Design review of the part built by this model. Coordinates are the model's own, in mm. Face numbers are marked on the shaded views. A direction names the side the tool comes from. Give positions to 0.01 mm unless a question says otherwise; leave off trailing zeros. Write each loop counter-clockwise with the first axis right and the second up, starting at its lowest first coordinate (ties: lowest second). Pieces come first, ordered by that corner, then holes. Notation, with made-up numbers: M 23,-9 L 45,-9 A31 cw 45,30 Z; hole C 83,-25 d6. An arc over 180 degrees is marked long. Use a Markdown table: item, result. Add a question column.
Autodesk Inventor part; units mm, degrees
ref_plane "YZ Plane" through (0, 0, 0) normal (1, 0, 0) x (0, 1, 0)
ref_plane "XZ Plane" through (0, 0, 0) normal (0, 1, 0) x (-1, 0, 0)
ref_plane "XY Plane" through (0, 0, 0) normal (0, 0, 1) x (1, 0, 0)
sketch "Sketch1" plane through (0, 0, 0) normal (0, 1, 0) x (-1, 0, 0)
  line L0 (0, 0) -> (19.1, 0)
  line L1 (19.1, 0) -> (19.1, -10)
  line L2 (19.1, -10) -> (0, -10)
  line L3 (0, -10) -> (0, 0)
  line L4 (12.55, -10) -> (6.55, -10)
  line L5 (6.55, -10) -> (6.55, -6)
  line L6 (6.55, -6) -> (12.55, -6)
  line L7 (12.55, -6) -> (12.55, -10)
  line L8 (0, 0) -> (-6, 0)
  line L9 (-6, 0) -> (-6, -17)
  line L10 (-6, -17) -> (0, -17)
  line L11 (0, -17) -> (0, 0)
  line L12 (19.1, 0) -> (25.1, 0)
  line L13 (25.1, 0) -> (25.1, -17)
  line L14 (25.1, -17) -> (19.1, -17)
  line L15 (19.1, -17) -> (19.1, 0)
  point P0 (9.55, -6)
  point P1 (9.55, 0)
  point P2 (6.55, -10)
  point P3 (0, -10)
  dimension "d0" = 6
  dimension "d1" = 19.1
  dimension "d2" = 4
  dimension "d3" = 10
  dimension "d6" = 6
  dimension "d7" = 6
  dimension "d8" = 17
  dimension "d20" = 7
extrude "Extrusion1" add sketch "Sketch1" along normal blind 10 contours L0 L1 L2 L7 L6 L5 L3 | L3 L11 L10 L9 L8 | L12 L13 L14 L15 L1
sketch "Sketch2" plane through (0, 0, 0) normal (0, -1, 0) x (1, 0, 0)
  line L0 (-25.1, 0) -> (6, 0)
  line L1 (-25.1, -17) -> (-25.1, 0)
  line L2 (-19.1, -17) -> (-25.1, -17)
  line L3 (-19.1, -10) -> (-19.1, -17)
  line L4 (-12.55, -10) -> (-19.1, -10)
  line L5 (-12.55, -6) -> (-12.55, -10)
  line L6 (-6.55, -6) -> (-12.55, -6)
  line L7 (-6.55, -10) -> (-6.55, -6)
  line L8 (0, -10) -> (-6.55, -10)
  line L9 (0, -17) -> (0, -10)
  line L10 (6, -17) -> (0, -17)
  line L11 (6, 0) -> (6, -17)
  line L12 (6, -17) -> (16, -17)
  line L13 (16, -17) -> (16, 10)
  line L14 (16, 10) -> (-35.1, 10)
  line L15 (-35.1, 10) -> (-35.1, -17)
  line L16 (-35.1, -17) -> (-25.1, -17)
  point P0 (0, 0)
  dimension "d9" = 10
  dimension "d10" = 10
  dimension "d11" = 10
extrude "Extrusion2" add sketch "Sketch2" against normal blind 2 contours L1 L16 L15 L14 L13 L12 L11 L0
chamfer "Chamfer1" distance 2 angle 45 7 edges at (-19.1, 10, -13.5) (-15.825, 10, -10) (-9.55, 10, -6) (-6.55, 10, -8) (0, 10, -13.5) (-3.275, 10, -10) (-12.55, 10, -8)
chamfer "Chamfer2" distance 2 angle 45 3 edges at (6, 10, -8.5) (-9.55, 10, 0) (-25.1, 10, -8.5)
properties part number "millmax_solder_rig"
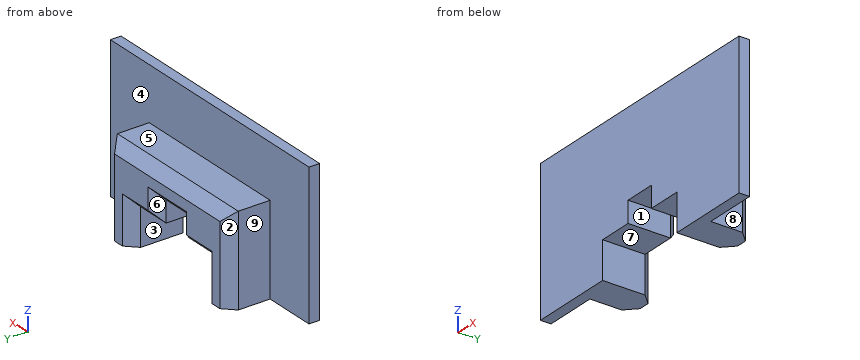
(1) Add section A-A on z = -10.5. Give the boundary of the cut face in (x, y), then the cut area to 3 significant figures.
(2) Add section B-B on y = 5.75. Give the boundary of the cut face in (x, z), then the cut area to 3 significant figures.
(3) For pin 1 (12 mm diameter, centred on x = -13.5, z = 7, fed in from +Y); pin 2 (2 mm diameter, centred on x = -1.5, z = -12, fed in from -Y); pin 3 (1.2 mm diameter, centred on y = 4, z = -8.5, fed in from +X); pin 4 (5 mm diameter, centred on x = -10, y = 7.5, fed in from +Z), all flat-tipped, find the tip position at first contact; note any pin that passes through.
(4) The part is to be moulded in two halves that separate along X. For the marked faces 1, 2, 3 and 4, say which applies: released by +X, released by -X, zero draft, split by the parting line, or undercut.
(5) Add section D-D on z = -2.5. Give the boundary of the cut face in (x, y), then the cut area to 3 significant figures.
(6) Machinability: for the marked faces 5, 6, 7, 8 and 9, which of the approach directions +Z, -Z, +X, -X, +Y, -Y give a long, thin tool a straight path to every point of the face, cutting with its end or side? Answer none if there is none.
(7) Wall thickness on L1, parallel to X at y = 5.75, z = -14.75; L2, parallel to X at y = 5.5, z = -9.75; L3, parallel to Z at x = -1.5, y = 2.75: over which ranges is each line inside the solid? List them lowest first.
(8) Add section C-C on x = -3.5. Give the boundary of the cut face in (y, z), then the cut area to 3 significant figures.
From the geometry:
| question | item | result |
|---|---|---|
| 1 | outline | M -35.1,0 L -19.1,0 L -19.1,8 L -21.1,10 L -23.1,10 L -25.1,8 L -25.1,2 L -35.1,2 Z; M 0,0 L 16,0 L 16,2 L 6,2 L 6,8 L 4,10 L 2,10 L 0,8 Z |
| 1 | area | 152 mm^2 |
| 2 | outline | M -25.1,-17 L -19.1,-17 L -19.1,-10 L -12.55,-10 L -12.55,-6 L -6.55,-6 L -6.55,-10 L 0,-10 L 0,-17 L 6,-17 L 6,0 L -25.1,0 Z |
| 2 | area | 371 mm^2 |
| 3 | pin 1 | stops at y = 2 |
| 3 | pin 2 | passes through |
| 3 | pin 3 | stops at x = 6 |
| 3 | pin 4 | stops at z = 0 |
| 4 | face 1 | undercut |
| 4 | face 2 | released by -X |
| 4 | face 3 | undercut |
| 4 | face 4 | zero draft |
| 5 | outline | M -35.1,0 L 16,0 L 16,2 L 6,2 L 6,8 L 4,10 L -23.1,10 L -25.1,8 L -25.1,2 L -35.1,2 Z |
| 5 | area | 347 mm^2 |
| 6 | face 5 | +Z, +X, -X, +Y |
| 6 | face 6 | -Z, +Y |
| 6 | face 7 | -Z, +Y, -Y |
| 6 | face 8 | +Z, -Z, +X, +Y |
| 6 | face 9 | +Z, -Z, -X, +Y |
| 7 | L1 | x = -25.1 to -19.1, 0 to 6 |
| 7 | L2 | x = -25.1 to -12.55, -6.55 to 6 |
| 7 | L3 | z = -10 to 0 |
| 8 | outline | M 0,-10 L 8,-10 L 10,-8 L 10,-2 L 8,0 L 2,0 L 2,10 L 0,10 Z |
| 8 | area | 116 mm^2 |
